Part model, mm, in its own coordinate system. A direction names the side the tool comes from. Coordinates: 2 decimals unless noted, no trailing zeros. Order: outer loops, then holes, each group sorted by start corner. A loop starts at its lowest first (then second) coordinate and runs counter-clockwise, first axis right, second up.
1) Cut at B-B (y = 3). List the corners of the cut face in (x, z).
2) Mould opens along X. For faces 4 (the flat face through (28, 17, 13)), 5 (the cylindrical face through (-2.385, 11.258, -8.59)), 6 (the flat face through (-30, 13, 12)) say: +X half, -X half, draft (parallel to the pull), parting line (faces both ways), or undercut.
3) Cut at C-C (z = 17.5). List the corners of the cut face in (x, y).
4) Cut at D-D (x = 25). List the corners of the cut face in (y, z).
5) Wall check: L1, parallel to X at y = 3, z = 17.5; L2, parallel to Z at x = -25, y = 26.5; L3, parallel to Z at x = 25, y = 6. Give the ranges that are in metal, low to high.
6) Pin check, flat tips, straight feed: pin 1 Ø1.8 at (x, z) = (25, 6) entering from +Y; pin 2 Ø3 at (x, z) = (19, -2.5) entering from -Y; pin 3 Ø1 at (x, z) = (-25.5, 12.5) entering from +Y; pin 4 Ø5 at (x, z) = (0.5, -6) entering from -Y. Stop position of each tip, or through.
7) Cut at A-A (x = -13.5). List the corners of the cut face in (y, z), and give its area (3 significant figures).
8) Tool access for faces 1 (the flat face through (-25, 8, 11.5)), 2 (the flat face through (0, 34, 1)), 3 (the flat face through (-0.14, 17.522, -0.934)): list every direction of +Z, -Z, +X, -X, +Y, -Y with a clear straight run to the whole face (end or side of a thin tool).
Autodesk Inventor part; units mm, degrees
ref_plane "Plan de construction2" through (0, 1.3303, -6.3624) normal (0, 0.2046669, -0.9788317) x (1, 0, 0)
ref_plane "Plan de construction3" through (30, 0, 0) normal (0, -0.9788317, -0.2046669) x (-1, 0, 0)
ref_plane "YZ Plane" through (0, 0, 0) normal (1, 0, 0) x (0, 1, 0)
sketch "Esquisse1" plane through (0, 0, 0) normal (0, 1, 0) x (-1, 0, 0)
  line L0 (0, 0) -> (30, 0)
  line L1 (30, 0) -> (30, 25)
  line L2 (30, 25) -> (-30, 25)
  line L3 (-30, 25) -> (-30, 0)
  line L4 (-30, 0) -> (0, 0)
  line L5 (0, 0) -> (0, 2.45)
  line L6 (0, 2.45) -> (28, 2.45)
  line L7 (28, 2.45) -> (28, 22.55)
  line L8 (28, 22.55) -> (-28, 22.55)
  line L9 (-28, 22.55) -> (-28, 2.45)
  line L10 (-28, 2.45) -> (0, 2.45)
  dimension "d0" = 30
  dimension "d1" = 25
  dimension "d2" = 60
  dimension "d3" = 30
  dimension "d4" = 2.45
  dimension "d5" = 28
  dimension "d7" = 20.1
  dimension "d8" = 56
extrude "Extrusion1" add sketch "Esquisse1" along normal blind 27
ref_plane "Plan de construction1" through (0, 0, 0) normal (0, 0.2046669, -0.9788317) x (1, 0, 0)
sketch "Esquisse10" plane through (0, 27, 0) normal (0, 1, 0) x (1, 0, 0)
  line L0 (-30, 0) -> (-30, -25)
  line L1 (30, -25) -> (30, 0)
  line L2 (-30, 0) -> (30, 0)
  line L3 (30, 0) -> (30, -2.45)
  line L4 (30, -2.45) -> (-30, -2.45)
  line L5 (-30, -2.45) -> (-30, 0)
  point P0 (0, 0)
  point P1 (30, 0)
  dimension "d67" = 2.45
extrude "Extrusion8" add sketch "Esquisse10" along normal blind 7
sketch "Esquisse2" plane through (0, 0, 0) normal (0, 0.2046669, -0.9788317) x (1, 0, 0)
  line L0 (0, 0) -> (0, -20)
  circle A0 centre (0, -20) radius 10
  circle A1 centre (0, -20) radius 11
  dimension "d12" = 20
  dimension "d13" = 20
  dimension "d14" = 22
extrude "Extrusion2" add sketch "Esquisse2" along normal blind 16.5
sketch "Esquisse3" plane through (0, 27, 0) normal (0, 1, 0) x (1, 0, 0)
  line L0 (-28, -22.55) -> (-28, -2.45)
  line L1 (28, -22.55) -> (-28, -22.55)
  line L2 (-28, -2.45) -> (28, -2.45)
  line L3 (28, -2.45) -> (28, -22.55)
  point P0 (0, 0)
extrude "Extrusion3" cut sketch "Esquisse3" against normal through all
ref_plane "Plan de construction2" through (0, 1.3303, -6.3624) normal (0, 0.2046669, -0.9788317) x (1, 0, 0)
sketch "Esquisse4" plane through (0, 1.3303, -6.3624) normal (0, 0.2046669, -0.9788317) x (1, 0, 0)
  circle A0 centre (0, -20) radius 10
  point P0 (0, 0)
extrude "Extrusion4" add sketch "Esquisse4" against normal blind 2
ref_plane "Plan de construction3" through (30, 0, 0) normal (0, -0.9788317, -0.2046669) x (-1, 0, 0)
sketch "Esquisse5" plane through (30, 0, 0) normal (0, -0.9788317, -0.2046669) x (-1, 0, 0)
  line L0 (41, 16.5) -> (19, 16.5)
  line L1 (30, 16.5) -> (30, 11.5)
  point P0 (30, 0)
  dimension "d23" = 5
hole "Perçage1" at (0, 2.3537, -11.2566) direction (0, 0.9788317, 0.2046669) diameter 4 end through all
sketch "Esquisse6" plane through (0, 0, 0) normal (0, -1, 0) x (1, 0, 0)
  line L0 (28, 2.45) -> (28, 22.55)
  line L1 (-28, 22.55) -> (-28, 2.45)
  line L2 (28, 22.55) -> (22, 22.55)
  line L3 (28, 22.55) -> (-28, 22.55)
  line L4 (22, 22.55) -> (22, 2.45)
  line L5 (22, 2.45) -> (28, 2.45)
  line L6 (-28, 22.55) -> (-22, 22.55)
  line L7 (-22, 22.55) -> (-22, 2.45)
  line L8 (-22, 2.45) -> (-28, 2.45)
  point P0 (0, 0)
  dimension "d31" = 6
  dimension "d32" = 6
extrude "Extrusion5" add sketch "Esquisse6" against normal blind 9
sketch "Esquisse7" plane through (0, 9, 0) normal (0, 1, 0) x (1, 0, 0)
  line L0 (-28, -22.55) -> (-28, -2.45)
  line L1 (-28, -12.5) -> (-25, -12.5)
  line L2 (-25, -12.5) -> (-25, -17.5)
  line L3 (-25, -12.5) -> (-25, -7.5)
  line L4 (28, -2.45) -> (28, -22.55)
  line L5 (28, -22.55) -> (28, -12.5)
  line L6 (28, -12.5) -> (25, -12.5)
  line L7 (25, -12.5) -> (25, -7.5)
  line L8 (22, -22.55) -> (22, -2.45)
  line L9 (25, -12.5) -> (25, -17.5)
  point P0 (0, 0)
  dimension "d35" = 3
  dimension "d36" = 5
  dimension "d37" = 5
  dimension "d38" = 3
  dimension "d39" = 5
  dimension "d41" = 5
hole "Perçage2" at (-25, 9, 17.5) at (-25, 9, 7.5) at (25, 9, 17.5) at (25, 9, 7.5) direction (0, -1, 0) diameter 3.242 depth 11.8 tip angle 118
sketch "Esquisse8" plane through (0, 9, 0) normal (0, 1, 0) x (1, 0, 0)
  line L0 (-22, -22.55) -> (-22, -2.45)
  line L1 (-28, -22.55) -> (-28, -2.45)
  line L2 (-28, -12.5) -> (-28, -11.5)
  line L3 (-28, -11.5) -> (-22, -11.5)
  line L4 (-28, -12.5) -> (-28, -13.5)
  line L5 (-28, -13.5) -> (-22, -13.5)
  line L6 (-22, -11.5) -> (-22, -13.5)
  line L7 (22, -2.45) -> (22, -22.55)
  line L8 (28, -2.45) -> (28, -22.55)
  line L9 (28, -22.55) -> (28, -12.5)
  line L10 (28, -12.5) -> (28, -11.5)
  line L11 (22, -11.5) -> (28, -11.5)
  line L12 (22, -11.5) -> (22, -13.5)
  line L13 (22, -13.5) -> (28, -13.5)
  point P0 (0, 0)
  point P1 (28, -12.5)
  point P2 (28, -13.5)
  dimension "d49" = 1
  dimension "d50" = 1
  dimension "d54" = 10.05
  dimension "d55" = 6
  dimension "d56" = 2
  dimension "d57" = 1
extrude "Extrusion6" cut sketch "Esquisse8" against normal blind 2
sketch "Esquisse11" plane through (0, 34, 0) normal (0, 1, 0) x (1, 0, 0)
  ellipse E0 centre (0, 31.4094) end of major axis (0, 85.1552) minor radius 11 (-8.5426, -2.45) -> (-7.9677, -5.6455) ccw
  ellipse E1 centre (0, -4.0933) end of major axis (11, -4.0933) minor radius 2.2513 (-7.9677, -5.6455) -> (7.9677, -5.6455) ccw
  ellipse E2 centre (0, 31.4094) end of major axis (0, 85.1552) minor radius 11 (7.9677, -5.6455) -> (8.5426, -2.45) ccw
  line L0 (-8.5426, -2.45) -> (8.5426, -2.45)
  point P0 (0, 0)
extrude "Extrusion9" cut sketch "Esquisse11" against normal blind 10
properties part number "Attache servomoteur"
Geometry check:
1. outline: (-30, 0) - (30, 0) - (30, 25) - (-30, 25) - close; hole circle Ø3.24 at (-25, 7.5); hole circle Ø3.24 at (-25, 17.5); hole (-22, 2.45) - (22, 2.45) - (22, 22.55) - (-22, 22.55) - close; hole circle Ø3.24 at (25, 7.5); hole circle Ø3.24 at (25, 17.5)
2. face 4: undercut
2. face 5: parting line
2. face 6: -X half
3. outline: (-30, 0) - (-26.62, 0) - (-26.62, 9) - (-28, 9) - (-28, 27) - (-30, 27) - close; (-23.38, 0) - (-22, 0) - (-22, 9) - (-23.38, 9) - close; (22, 0) - (23.38, 0) - (23.38, 9) - (22, 9) - close; (26.62, 0) - (30, 0) - (30, 27) - (28, 27) - (28, 9) - (26.62, 9) - close
4. outline: (0, 0) - (34, 0) - (34, 2.45) - (9, 2.45) - (9, 5.88) - (0, 5.88) - close; (0, 9.12) - (9, 9.12) - (9, 11.5) - (7, 11.5) - (7, 13.5) - (9, 13.5) - (9, 15.88) - (0, 15.88) - close; (0, 19.12) - (9, 19.12) - (9, 22.55) - (27, 22.55) - (27, 25) - (0, 25) - close
5. L1: x = -30 to -26.62, -23.38 to -22, 22 to 23.38, 26.62 to 30
5. L2: z = 0 to 2.45, 22.55 to 25
5. L3: z = 0 to 5.88, 9.12 to 15.88, 19.12 to 25
6. pin 1: stops at y = 9
6. pin 2: passes through
6. pin 3: stops at y = 7
6. pin 4: stops at y = 9.93
7. outline: (0, 0) - (34, 0) - (34, 2.45) - (0, 2.45) - close; (0, 22.55) - (27, 22.55) - (27, 25) - (0, 25) - close
7. area: 149 mm2
8. face 1: +Y
8. face 2: +Z, -Z, +X, -X, +Y
8. face 3: none
